Can you work these out from the model? Positions are in its coordinate system, mm. Give positions to 0.01 mm unless a question says otherwise; leave off trailing zeros. Order: outer loops, then holes, each group sorted by start corner. A loop starts at its lowest first (then second) coordinate and runs counter-clockwise, first axis right, second up.
Item 1: If I drill on line 1 along Y through (x, z) = (321, 17); line 2 along Y through (x, z) = (285, 15.25); line 3 along Y through (x, z) = (508, 9), over which ranges is the centre line in solid material (lowest first)?
Item 2: I want a section at D-D, the plane x = 432. Write out the boundary of the cut face in (y, z).
Item 3: I want a section at C-C, the plane y = -103. Write out the boundary of the cut face in (x, z), then the cut area to 3 significant figures.
Item 4: I'm going to push flat-ended pins straight in: pin 1 Ø1.7 at (y, z) = (-124, 14) entering from -X; pin 2 Ø0.6 at (y, z) = (124, 13) entering from -X; pin 3 Ø10 at (y, z) = (17, 4) entering from +X. Where does each tip first touch, or does it pass through?
Item 5: I want a section at B-B, the plane z = 7.5. Count the separate pieces of the cut face and the enclosed holes in it, then the cut area to 3 significant figures.
Item 6: I want a section at A-A, the plane x = 179.5. Write out the boundary of the cut face in (y, z).
Autodesk Inventor part; units mm, degrees
ref_plane "Work Plane1" through (0, 0, 0) normal (0, 0, 1) x (1, 0, 0)
ref_plane "YZ Plane" through (0, 0, 0) normal (1, 0, 0) x (0, 1, 0)
ref_plane "XZ Plane" through (0, 0, 0) normal (0, 1, 0) x (-1, 0, 0)
ref_plane "Work Plane1" through (0, 0, 0) normal (0, 0, 1) x (1, 0, 0)
sketch "Sketch1" plane through (0, 0, 0) normal (0, 0, 1) x (1, 0, 0)
  line L0 (73.4542, 120.707) -> (75.2544, 119.6677)
  arc A0 (73.4542, 120.707) -> (70.7046, 122.2945) centre (72.0794, 121.5007) ccw
  line L1 (68.9044, 123.3338) -> (70.7046, 122.2945)
  line L2 (68.9044, 125.4125) -> (68.9044, 123.3338)
  arc A1 (68.9044, 125.4125) -> (68.9044, 128.5875) centre (68.9044, 127) ccw
  line L3 (68.9044, 130.6662) -> (68.9044, 128.5875)
  line L4 (70.7046, 131.7055) -> (68.9044, 130.6662)
  arc A2 (70.7046, 131.7055) -> (73.4542, 133.293) centre (72.0794, 132.4993) ccw
  line L5 (75.2544, 134.3323) -> (73.4542, 133.293)
  line L6 (77.0546, 133.293) -> (75.2544, 134.3323)
  arc A3 (77.0546, 133.293) -> (79.8042, 131.7055) centre (78.4294, 132.4993) ccw
  line L7 (81.6044, 130.6662) -> (79.8042, 131.7055)
  line L8 (81.6044, 128.5875) -> (81.6044, 130.6662)
  arc A4 (81.6044, 128.5875) -> (81.6044, 125.4125) centre (81.6044, 127) ccw
  line L9 (81.6044, 123.3338) -> (81.6044, 125.4125)
  line L10 (79.8042, 122.2945) -> (81.6044, 123.3338)
  arc A5 (79.8042, 122.2945) -> (77.0546, 120.707) centre (78.4294, 121.5007) ccw
  line L11 (75.2544, 119.6677) -> (77.0546, 120.707)
  circle A6 centre (75.2544, 127) radius 2.9337
  line L12 (73.4542, -133.293) -> (75.2544, -134.3323)
  arc A7 (73.4542, -133.293) -> (70.7046, -131.7055) centre (72.0794, -132.4993) ccw
  line L13 (68.9044, -130.6662) -> (70.7046, -131.7055)
  line L14 (68.9044, -128.5875) -> (68.9044, -130.6662)
  arc A8 (68.9044, -128.5875) -> (68.9044, -125.4125) centre (68.9044, -127) ccw
  line L15 (68.9044, -123.3338) -> (68.9044, -125.4125)
  line L16 (70.7046, -122.2945) -> (68.9044, -123.3338)
  arc A9 (70.7046, -122.2945) -> (73.4542, -120.707) centre (72.0794, -121.5007) ccw
  line L17 (75.2544, -119.6677) -> (73.4542, -120.707)
  line L18 (77.0546, -120.707) -> (75.2544, -119.6677)
  arc A10 (77.0546, -120.707) -> (79.8042, -122.2945) centre (78.4294, -121.5007) ccw
  line L19 (81.6044, -123.3338) -> (79.8042, -122.2945)
  line L20 (81.6044, -125.4125) -> (81.6044, -123.3338)
  arc A11 (81.6044, -125.4125) -> (81.6044, -128.5875) centre (81.6044, -127) ccw
  line L21 (81.6044, -130.6662) -> (81.6044, -128.5875)
  line L22 (79.8042, -131.7055) -> (81.6044, -130.6662)
  arc A12 (79.8042, -131.7055) -> (77.0546, -133.293) centre (78.4294, -132.4993) ccw
  line L23 (75.2544, -134.3323) -> (77.0546, -133.293)
  circle A13 centre (75.2544, -127) radius 2.9337
  line L24 (75.2544, -127) -> (513.2774, 0) construction
  line L25 (106.8774, 406.4) -> (106.8774, -406.4)
  line L26 (106.8774, 0) -> (513.2774, 0)
  line L27 (513.2774, 0) -> (75.2544, 127) construction
  line L28 (75.2544, 127) -> (68.1812, 102.6047) construction
  line L29 (75.2544, 127) -> (82.3275, 151.3953) construction
  line L30 (75.2544, 127) -> (50.8591, 134.0732) construction
  line L31 (82.3275, 151.3953) -> (57.9322, 158.4684)
  line L32 (57.9322, 158.4684) -> (50.8591, 134.0732)
  line L33 (50.8591, 134.0732) -> (43.7859, 109.6779)
  line L34 (43.7859, 109.6779) -> (68.1812, 102.6047)
  line L35 (82.3275, 151.3953) -> (513.2774, 26.4461)
  line L36 (68.1812, 102.6047) -> (164.7505, 74.6055)
  line L37 (538.647, 19.0904) -> (533.1119, 0)
  line L38 (524.5007, 29.7002) -> (513.2774, 26.4461)
  line L39 (43.7859, -109.6779) -> (57.9322, -158.4684)
  line L40 (57.9322, -158.4684) -> (513.2774, -26.4461)
  line L41 (538.647, -19.0904) -> (533.1119, 0)
  line L42 (266.3505, 45.1477) -> (379.9952, 12.1976)
  line L43 (164.7505, 74.6055) -> (266.3505, 45.1477)
  line L44 (164.7505, -74.6055) -> (43.7859, -109.6779)
  line L45 (266.3505, -45.1477) -> (164.7505, -74.6055)
  line L46 (379.9952, -12.1976) -> (266.3505, -45.1477)
  line L47 (379.9952, 12.1976) -> (513.2774, -26.4461) construction
  line L48 (513.2774, -26.4461) -> (524.5007, -29.7002)
  line L49 (513.2774, 26.4461) -> (526.5609, 22.5947)
  line L50 (513.2774, 26.4461) -> (379.9952, -12.1976) construction
  line L51 (513.2774, -26.4461) -> (538.647, -19.0904)
  arc A14 (379.9952, -12.1976) -> (379.9952, 12.1976) centre (376.4586, 0) ccw
  line L52 (526.5609, -22.5947) -> (524.5007, -29.7002)
  line L53 (526.5609, 22.5947) -> (538.647, 19.0904)
  line L54 (533.1119, 0) -> (526.5609, -22.5947)
  line L55 (533.1119, 0) -> (524.5007, 29.7002)
  point P0 (0, 0)
  dimension "d0" = 406.4
  dimension "d1" = 25.4
  dimension "d2" = 25.4
  dimension "d3" = 25.4
  dimension "d4" = 19.05
  dimension "d7" = 25.4
  dimension "d8" = 25.4
  dimension "d9" = 25.4
  dimension "d10" = 19.05
  dimension "d15" = 12.7
extrude "Extrusion2" add sketch "Sketch1" along normal blind 19.05 contours L35 L49 L55 L54 L51 L40 L25 L44 L45 L46 A14 L42 L43 L36 | L25 L36 L34 L33 L32 L31 L35 | L25 L40 L39 L44
properties part number "aFrameBase"
Results list:
1. line 1: y = -82.19 to -29.3, 29.3 to 82.19
1. line 2: y = -92.63 to -39.74, 39.74 to 92.63
1. line 3: y = -27.98 to 27.98
2. outline: (-50.01, 0) - (50.01, 0) - (50.01, 19.05) - (-50.01, 19.05) - close
3. outline: (66.82, 0) - (249.24, 0) - (249.24, 19.05) - (66.82, 19.05) - close
3. area: 3,480 mm2
4. pin 1: stops at x = 47.69
4. pin 2: stops at x = 47.85
4. pin 3: stops at x = 529.63
5. separate pieces: 1
5. enclosed holes: 2
5. area: 47,400 mm2
6. outline: (-123.22, 0) - (-70.33, 0) - (-70.33, 19.05) - (-123.22, 19.05) - close; (70.33, 0) - (123.22, 0) - (123.22, 19.05) - (70.33, 19.05) - close
